```python
from build123d import *

# Parameters (mm, degrees)
SKETCH_W        = 150
SKETCH_H        = 130
SKETCH_R        = 8
SKETCH_R_2      = 1.75
SKETCH_W_2      = 110
SKETCH_H_2      = 68
PAD_DEPTH       = 3
SKETCH002_W     = 132
SKETCH002_H     = 77
POCKET001_DEPTH = 2.5
SKETCH007_W     = 5.5
SKETCH007_H     = 6
SKETCH007_R     = 2
PAD002_DEPTH    = 6
PAD003_DEPTH    = 10
SKETCH010_R     = 1.75
POCKET002_DEPTH = 6
SKETCH011_R     = 1.75
POCKET003_DEPTH = 7.5
SKETCH012_R     = 1.75
POCKET004_DEPTH = 7.5
SKETCH014_W     = 0.7
SKETCH014_H     = 6.545228
PAD004_DEPTH    = 2.5
SKETCH015_R     = 3.05
POCKET_DEPTH    = 13.001
SKETCH016_W     = 0.7
SKETCH016_H     = 6.545228
PAD005_DEPTH    = 2.5


with BuildPart() as part:
    # Sketch → Pad (new body)
    with BuildSketch(Plane.XY):
        with Locations((-75, -5)):
            Rectangle(SKETCH_W, SKETCH_H)
        with Locations((-23.386462, -40.5)):
            Circle(SKETCH_R, mode=Mode.SUBTRACT)
        with Locations((-141, 45)):
            Circle(SKETCH_R_2, mode=Mode.SUBTRACT)
        with Locations((-141, -26)):
            Circle(SKETCH_R_2, mode=Mode.SUBTRACT)
        with Locations((-13.5, 45)):
            Circle(SKETCH_R_2, mode=Mode.SUBTRACT)
        with Locations((-13.5, -26)):
            Circle(SKETCH_R_2, mode=Mode.SUBTRACT)
        with Locations((-4, 56)):
            Circle(SKETCH_R_2, mode=Mode.SUBTRACT)
        with Locations((-4, -66)):
            Circle(SKETCH_R_2, mode=Mode.SUBTRACT)
        with Locations((-77, 11)):
            Rectangle(SKETCH_W_2, SKETCH_H_2, mode=Mode.SUBTRACT)
    extrude(amount=PAD_DEPTH)

    # Sketch002 → Pocket001 (cut)
    with BuildSketch(Plane.XY.offset(3.5)):
        with Locations((-77, 9.5)):
            Rectangle(SKETCH002_W, SKETCH002_H)
    extrude(amount=-POCKET001_DEPTH, mode=Mode.SUBTRACT)

    # Sketch007 → Pad002 (join)
    with BuildSketch(Plane.XY):
        with Locations((-141.25, 45)):
            Rectangle(SKETCH007_W, SKETCH007_H)
        with Locations((-141.5, 45)):
            Circle(SKETCH007_R, mode=Mode.SUBTRACT)
        with Locations((-13.75, 45)):
            Rectangle(SKETCH007_W, SKETCH007_H)
        with Locations((-13.5, 45)):
            Circle(SKETCH007_R, mode=Mode.SUBTRACT)
        with Locations((-13.75, -26)):
            Rectangle(SKETCH007_W, SKETCH007_H)
        with Locations((-13.5, -26)):
            Circle(SKETCH007_R, mode=Mode.SUBTRACT)
        with Locations((-141.25, -26)):
            Rectangle(SKETCH007_W, SKETCH007_H)
        with Locations((-141.5, -26)):
            Circle(SKETCH007_R, mode=Mode.SUBTRACT)
    extrude(amount=PAD002_DEPTH)

    # Sketch003 (on DatumPlane) → Pad003 (join)
    with BuildSketch(Plane.XY.offset(3)):
        Polygon((-20, 60), (-150, 60), (-150, -60), (-20, -60), (-20, -57), (-147, -57), (-147, 57), (-20, 57), align=None)
    extrude(amount=PAD003_DEPTH)

    # Sketch010 → Pocket002 (cut)
    with BuildSketch(Plane.XZ.offset(60)):
        with Locations((-125, 9.5)):
            Circle(SKETCH010_R)
        with Locations((-25, 9.5)):
            Circle(SKETCH010_R)
        with Locations((-75, 9.5)):
            Circle(SKETCH010_R)
    extrude(amount=-POCKET002_DEPTH, mode=Mode.SUBTRACT)

    # Sketch011 → Pocket003 (cut, symmetric)
    with BuildSketch(Plane.XZ.offset(-60)):
        with Locations((-75, 9.5)):
            Circle(SKETCH011_R)
        with Locations((-25, 9.5)):
            Circle(SKETCH011_R)
        with Locations((-125, 9.5)):
            Circle(SKETCH011_R)
    extrude(amount=POCKET003_DEPTH, both=True, mode=Mode.SUBTRACT)

    # Sketch012 (on DatumPlane) → Pocket004 (cut, symmetric)
    with BuildSketch(Plane.YZ.offset(-150)):
        with Locations((0, 9.5)):
            Circle(SKETCH012_R)
        with Locations((50, 9.5)):
            Circle(SKETCH012_R)
        with Locations((-50, 9.5)):
            Circle(SKETCH012_R)
    extrude(amount=POCKET004_DEPTH, both=True, mode=Mode.SUBTRACT)

    # Sketch014 → Pad004 (join)
    with BuildSketch(Plane.XY):
        with Locations((-31.036462, -40.5)):
            Rectangle(SKETCH014_W, SKETCH014_H)
    extrude(amount=PAD004_DEPTH)

    # Sketch015 (on Face4 of Pad004) → Pocket (cut, through all)
    with BuildSketch(Plane(origin=(0, 0, 0), x_dir=(1, 0, 0), z_dir=(0, 0, -1))):
        with Locations((-48.386462, 40.5)):
            Circle(SKETCH015_R)
        with Locations((-73.386462, 40.5)):
            Circle(SKETCH015_R)
        with Locations((-98.386462, 40.5)):
            Circle(SKETCH015_R)
    extrude(amount=-POCKET_DEPTH, mode=Mode.SUBTRACT)

    # Sketch016 (on Face4 of Pocket) → Pad005 (join)
    with BuildSketch(Plane(origin=(0, 0, 0), x_dir=(1, 0, 0), z_dir=(0, 0, -1))):
        with Locations((-15.736462, 40.5)):
            Rectangle(SKETCH016_W, SKETCH016_H)
    extrude(amount=-PAD005_DEPTH)


solid = part.part
```
Design review of the part built by this model. Coordinates are the model's own, in mm. A direction names the side the tool comes from. Coordinates: 2 decimals unless noted, no trailing zeros. Order: outer loops, then holes, each group sorted by start corner. A loop starts at its lowest first (then second) coordinate and runs counter-clockwise, first axis right, second up. Notation, with made-up numbers: M 43,16.5 L 51,16.5 A9 ccw 51,31.5 Z; hole C -22,-21.75 d10. An arc over 180 degrees is marked long. Answer as a JSON object with one key per item and string values. Group by question number.
1) Add section C-C, the plane x = -87.5. Write out the cut boundary in (y, z).
2) Add section A-A, the plane x = -13.5. Write out the cut boundary in (y, z).
3) Tool access review of faces 5 (the flat face through (-139, 45, 6)), 6 (the flat face through (-14, 48, 4)), 7 (the cylindrical face through (-15.1, -27.2, 3.5)): name each direction out of +Z, -Z, +X, -X, +Y, -Y from which nothing blocks a thin tool from reaching the whole face with its end or side.
4) Add section D-D, the plane z = 9.5. Count the separate pieces of the cut face and the enclosed holes in it, then the cut area to 3 significant figures.
5) Add section B-B, the plane y = 16. Write out the cut boundary in (x, z).
6) Wall thickness on L1, parallel to Y at x = -141.5, z = 3.45; L2, parallel to Y at x = -13.5, z = 4.1; L3, parallel to Y at x = -69, z = 12.5: over which ranges is each line inside the solid? List them lowest first.
7) Mouldability with a two-part tool opening along X and no side actions: class faces 1 (the cylindrical face through (-139.592, -25.399, 3.625)), 2 (the flat face through (-20, -59, 8)), 3 (the flat face through (-77, -25, 1)), 4 (the flat face through (-76, -70, 1)) as pulls with the +X half, pulls with the -X half, needs draft (parallel to the pull), parting line crosses it, or undercut.
8) For pin 1 (6 mm diameter, centred on x = -141.5, y = -27, fed in from +Z); pin 2 (2 mm diameter, centred on x = -132, z = 8.5, fed in from -Y); pin 3 (5 mm diameter, centred on y = -28, z = 6, fed in from +X), all flat-tipped, find the tip position at first contact; note any pin that passes through.
Computed values:
{
 "1": {"outline": "M -70,0 L -23,0 L -23,1 L -29,1 L -29,3 L -57,3 L -57,13 L -60,13 L -60,3 L -70,3 Z; M 45,0 L 60,0 L 60,13 L 57,13 L 57,3 L 48,3 L 48,1 L 45,1 Z"},
 "2": {"outline": "M -70,0 L -27.75,0 L -27.75,1 L -28,1 L -28,6 L -29,6 L -29,3 L -70,3 Z; M -24.25,0 L 43.25,0 L 43.25,1 L 43,1 L 43,6 L 42,6 L 42,1 L -23,1 L -23,6 L -24,6 L -24,1 L -24.25,1 Z; M 46.75,0 L 60,0 L 60,3 L 48,3 L 48,6 L 47,6 L 47,1 L 46.75,1 Z"},
 "3": {"face 5": "+Z, +X", "face 6": "+Z, +X, +Y", "face 7": "+Z"},
 "4": {"separate pieces": "10", "enclosed holes": "0", "area": "1,030 mm^2"},
 "5": {"outline": "M -150,0 L -132,0 L -132,1 L -143,1 L -143,3 L -147,3 L -147,13 L -150,13 Z; M -22,0 L 0,0 L 0,3 L -11,3 L -11,1 L -22,1 Z"},
 "6": {"L1": "y = -60 to -57, -29 to -28, -24 to -23, 42 to 43, 47 to 48, 57 to 60", "L2": "y = -29 to -28, -24 to -23, 42 to 43, 47 to 48", "L3": "y = -60 to -57, 57 to 60"},
 "7": {"face 1": "undercut", "face 2": "pulls with the +X half", "face 3": "undercut", "face 4": "needs draft"},
 "8": {"pin 1": "stops at z = 6", "pin 2": "stops at y = -60", "pin 3": "stops at x = -11"}
}
